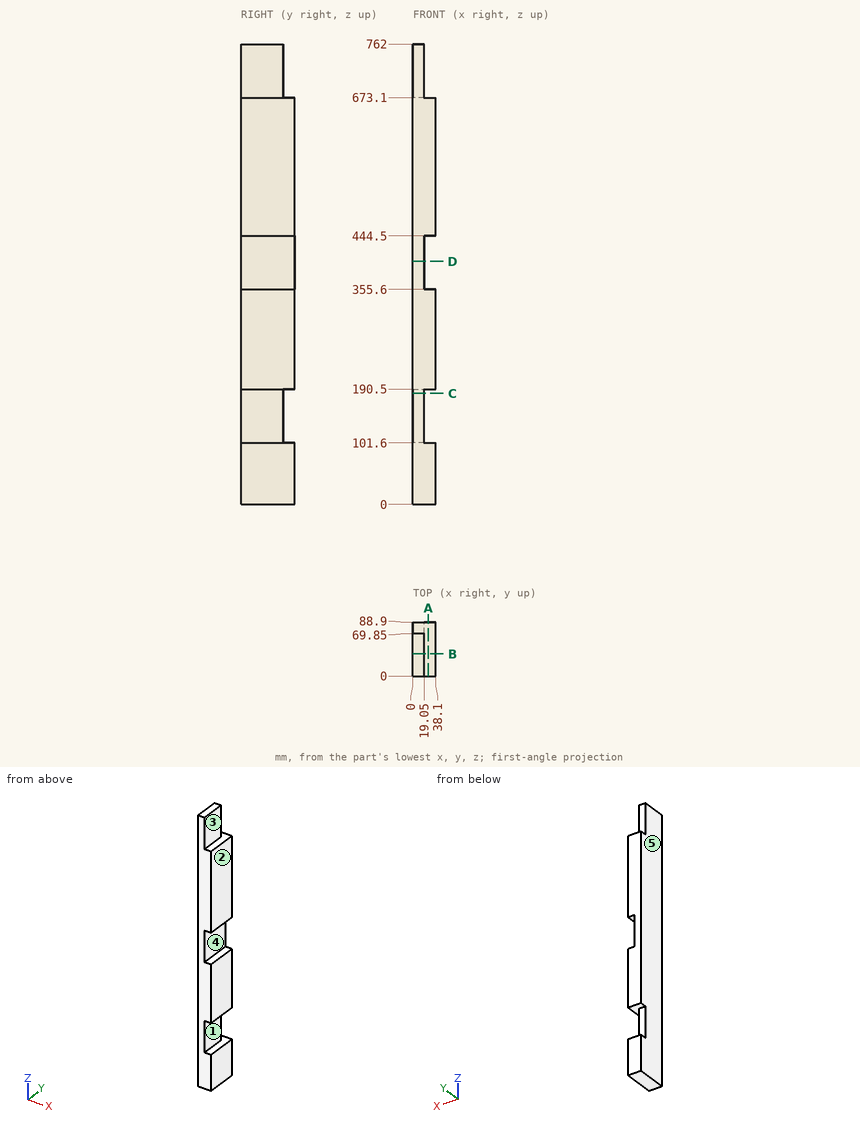
Verification items for this drawing (mm, ordinates from the low corner). A direction names the side the tool comes from. Coordinates: 2 decimals unless noted, no trailing zeros. Order: outer loops, then holes, each group sorted by start corner. A loop starts at its lowest first (then second) coordinate and runs counter-clockwise, first axis right, second up. Notation, with made-up numbers: (-13, 65) -> (9, 65) arc R14 cw to (9, 77) -> close; hole circle Ø8 at (-16.75, 59). An arc over 180 degrees is marked (long way). Answer as CSV lines item,"result". Start each with the question number.
1) Cross-section at B-B, the plane y = 36.5. Record the boundary of the cut face in (x, z), then the cut area to 3 significant figures.
2) Set-up check for the marked faces 1, 2 and 3: record each of +Z, -Z, +X, -X, +Y, -Y from which the full face is reachable in a straight line by a thin tool's end or side.
3) Cross-section at D-D, the plane z = 402. Record the boundary of the cut face in (x, y).
4) Gauge pin test, flat ends, axial feed: pin 1 Ø10 at (y, z) = (68, 121.5) entering from +X; pin 2 Ø5.5 at (x, z) = (9, 156.5) entering from +Y; pin 3 Ø4 at (x, y) = (10.5, 79.5) entering from +Z. Record the tip position at first contact, or that the pin passes through.
5) Cross-section at A-A, the plane x = 25.5. Record the boundary of the cut face in (y, z).
6) Release check for a two-part mould opening along Z. For the marked faces 4 and 5 record: released by +Z, released by -Z, zero draft, split by the parting line, or undercut.
7) Cross-section at C-C, the plane z = 183.5. Record the boundary of the cut face in (x, y), then the cut area to 3 significant figures.
8) Material ranges on L1, parallel to Z at x = 36, y = 65.5; L2, parallel to Z at x = 18.5, y = 76.5; L3, parallel to X at y = 9.5, z = 408.5, recorded low to high. Write a range as [from, to].
Conclusion:
1,outline,"(0, 0) -> (38.1, 0) -> (38.1, 101.6) -> (19.05, 101.6) -> (19.05, 190.5) -> (38.1, 190.5) -> (38.1, 355.6) -> (19.05, 355.6) -> (19.05, 444.5) -> (38.1, 444.5) -> (38.1, 673.1) -> (19.05, 673.1) -> (19.05, 762) -> (0, 762) -> close"
1,area,"24,000 mm²"
2,face 1,"+X, +Y, -Y"
2,face 2,"+Z, -Z, +X, +Y, -Y"
2,face 3,"+Z, +X, +Y, -Y"
3,outline,"(0, 0) -> (19.05, 0) -> (19.05, 88.9) -> (0, 88.9) -> close"
4,pin 1,"stops at x = 19.05"
4,pin 2,"stops at y = 69.85"
4,pin 3,"stops at z = 673.1"
5,outline,"(0, 0) -> (88.9, 0) -> (88.9, 101.6) -> (0, 101.6) -> close; (0, 190.5) -> (88.9, 190.5) -> (88.9, 355.6) -> (0, 355.6) -> close; (0, 444.5) -> (88.9, 444.5) -> (88.9, 673.1) -> (0, 673.1) -> close"
6,face 4,"undercut"
6,face 5,"zero draft"
7,outline,"(0, 0) -> (19.05, 0) -> (19.05, 69.85) -> (0, 69.85) -> close"
7,area,"1,330 mm²"
8,L1,"z = [0, 101.6], [190.5, 355.6], [444.5, 673.1]"
8,L2,"z = [0, 101.6], [190.5, 673.1]"
8,L3,"x = [0, 19.05]"
